Autodesk Inventor part; units mm, degrees
ref_plane "Plano de trabalho1" through (-14.4853, -144.1477, 29.69) normal (0, 0, -1) x (0, 1, 0)
ref_plane "YZ Plane" through (0, 0, 0) normal (1, 0, 0) x (0, 1, 0)
ref_plane "XZ Plane" through (0, 0, 0) normal (0, 1, 0) x (-1, 0, 0)
sketch "Esboço1" plane through (0, 0, 0) normal (0, 0, 1) x (1, 0, 0)
  line L0 (4.9347, -7.2977) -> (-6.5153, -7.2977)
  line L1 (4.9347, -7.2977) -> (4.9347, 10.1323)
  line L2 (4.9347, 10.1323) -> (2.5947, 10.1323)
  line L3 (2.5947, 10.1323) -> (-0.1453, 0.6423)
  line L4 (-0.1453, 0.6423) -> (-0.1453, -1.2977)
  arc A0 (-2.7953, -1.2977) -> (-0.1453, -1.2977) centre (-1.4703, -1.2977) ccw
  line L5 (-2.7953, -1.2977) -> (-2.7953, 2.6323)
  line L6 (-2.7953, 2.6323) -> (-6.5153, 2.6323)
  line L7 (-6.5153, 2.6323) -> (-6.5153, -7.2977)
  line L8 (-7.4703, 4.7023) -> (4.5297, 4.7023)
  line L9 (4.5297, 4.7023) -> (4.5297, -7.2977)
  line L10 (4.5297, -7.2977) -> (-7.4703, -7.2977)
  line L11 (-7.4703, -7.2977) -> (-7.4703, 4.7023)
  line L12 (-7.4703, 4.7023) -> (4.5297, -7.2977) construction
  line L13 (4.5297, 4.7023) -> (-7.4703, -7.2977) construction
  point P0 (0, 0)
  dimension "d0" = 12
  dimension "d1" = 12
ref_plane "Plano de trabalho1" through (-14.4853, -144.1477, 29.69) normal (0, 0, -1) x (0, 1, 0)
extrude "Extrusão1" add sketch "Esboço1" along normal up to surface (29.69 mm away) contours L0 L7 L6 L5 A0 L4 L3 L8 L9 | L10 L11 L8 L3 L4 A0 L5 L6 L7
sketch "Esboço3" plane through (0, 0, 0) normal (0, 0, -1) x (-1, 0, 0)
  line L0 (-4.5297, 4.7023) -> (7.4703, 4.7023)
  line L1 (7.4703, -7.2977) -> (-4.5297, -7.2977)
  line L2 (-4.5297, -7.2977) -> (-4.5297, 4.7023) construction
  line L3 (-4.5297, 4.7023) -> (7.4703, -7.2977) construction
  line L4 (7.4703, 4.7023) -> (-4.5297, -7.2977) construction
  circle A0 centre (1.4703, -1.2977) radius 3 construction
  dimension "d13" = 6
hole "Furo2" at (-1.4703, -1.2977, 0) direction (0, 0, 1) diameter 3.242 depth 12 tip angle 118
sketch "Esboço5" plane through (-7.4703, 4.7023, 29.69) normal (0, 0, 1) x (1, 0, 0)
  circle A0 centre (6, -6) radius 1.621
  circle A1 centre (6, -6) radius 3.7537 construction
hole "Furo3" at (-1.4703, -1.2977, 29.69) direction (0, 0, -1) diameter 3.242 depth 12 tip angle 118
properties part number "espassador_soprador" material "Alumínio 6061"
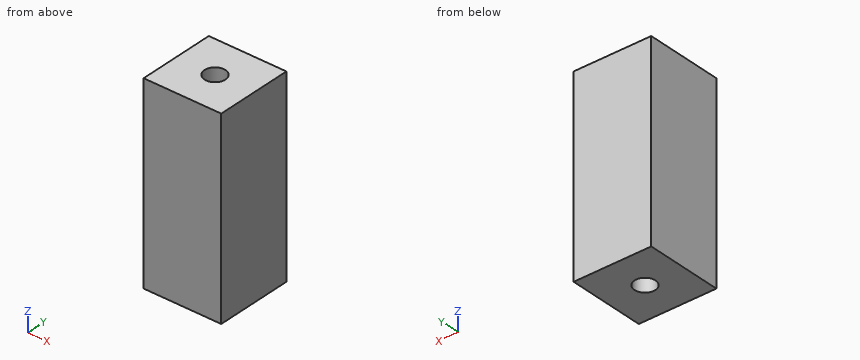
Geometry check sheet. Reference: the model listing, model coordinates, mm. Coordinates: 2 decimals unless noted, no trailing zeros. Order: outer loops, then holes, each group sorted by start corner. A loop starts at its lowest first (then second) coordinate and runs counter-clockwise, first axis right, second up.
Item 1: Depth check by flat-ended pin: pin 1 (1.9 mm diameter, centred on x = -1.47, y = -1.3, fed in from -Z). Enter the tip coordinate at first touch or a pass-through.
Item 2: Section check A-A (z = 24.25). Enter the section's corners in (x, y).
Item 3: Scan lines: line 1 along X through (y, z) = (-1, 18.75); line 2 along Y through (x, z) = (-1, 24.5); line 3 along X through (y, z) = (-2.75, 20). Record each from-to range of solid material in increasing order.
Check sheet entries:
1. pin 1: stops at z = 12.4
2. outline: (-7.47, -7.3) - (4.53, -7.3) - (4.53, 4.7) - (-7.47, 4.7) - close; hole circle Ø3.24 at (-1.47, -1.3)
3. line 1: x = -7.47 to -3.06, 0.12 to 4.53
3. line 2: y = -7.3 to -2.85, 0.25 to 4.7
3. line 3: x = -7.47 to -2.19, -0.75 to 4.53
